Input: part model. Units: mm. Frame: model coordinates. A direction names the side the tool comes from. Round coordinates to 2 decimals unless told otherwise and drop trailing zeros. Order: outer loops, then holes, each group sorted by start corner. A loop starts at its lowest first (then second) coordinate and runs counter-clockwise, first axis right, second up. Notation, with made-up numbers: (68, -32) -> (121, -32) arc R21 cw to (121, -1) -> close; hole circle Ø6 at (66, 63). An arc over 180 degrees is marked (long way). Answer as CSV lines item,"result". Start each with the question number.
1) Access query for faces 4 (the face through (31.056, 27.135, 5.07)), 5 (the face through (-10, -33, 10)), 6 (the face through (5.961, -26.846, 14.058)). Directions: +Z, -Z, +X, -X, +Y, -Y. A direction counts if a zero-diameter tool reaches every point of the face in a straight line with its end or side. Return the directions, or none.
2) Section query D-D, the plane z = 15.5. Output: boundary loops of the cut face in (x, y).
3) First-contact query: P1, Ø12, axis at x = 18, y = -30, coming from the -Z side; P2, Ø5.5, axis at x = 28.28, y = -28.28, coming from the +Z side; P3, Ø7, axis at x = -28.28, y = 28.28, coming from the +Z side; P4, Ø10, axis at y = 4.5, z = 27, coming from the +X side. Flat tips, straight axial feed; report the tip coordinate or a pass-through.
4) Section query A-A, the plane y = 0. State how many separate pieces and enclosed holes the cut face has, and give its area (4 significant figures).
5) Line query: L1, parallel to Z at x = 37.5, y = 18; L2, parallel to X at y = 8, z = 30.5. Output: solid intervals per line, ascending.
6) Mould query, pull axis Y, two halves, no side actions, for faces 1 (the face through (18.28, 28.67, 21.09)), 2 (the face through (0, 43, 5)), 3 (the face through (-1, -29, 0)). Classes: +Y half, -Y half, draft (parallel to the pull), parting line (faces both ways), or undercut.
```python
from build123d import *

# Parameters (mm, degrees)
SKETCH_1_R          = 45
EXTRUDE_1_DEPTH     = 10
SKETCH_2_R          = 34
EXTRUDE_2_DEPTH     = 23
SKETCH_4_R          = 25
CUT_EXTRUDE_1_DEPTH = 70
SKETCH_5_R          = 27.5
CUT_EXTRUDE_2_DEPTH = 28
SKETCH_6_R          = 3
CUT_EXTRUDE_3_DEPTH = 25
CHAMFER_1_SIZE      = 0.5


with BuildPart() as part:
    # 草图1 → 拉伸1 (new body)
    with BuildSketch(Plane.XY):
        Circle(SKETCH_1_R)
    extrude(amount=EXTRUDE_1_DEPTH)

    # 草图2 → 拉伸2 (add)
    with BuildSketch(Plane.XY.offset(10)):
        Circle(SKETCH_2_R)
    extrude(amount=EXTRUDE_2_DEPTH)

    # 草图4 → 切除-拉伸1 (cut)
    with BuildSketch(Plane.XY.offset(33)):
        Circle(SKETCH_4_R)
    extrude(amount=-CUT_EXTRUDE_1_DEPTH, mode=Mode.SUBTRACT)

    # 草图5 → 切除-拉伸2 (cut)
    with BuildSketch(Plane(origin=(0, 0, 0), x_dir=(-1, 0, 0), z_dir=(0, 0, -1))):
        Circle(SKETCH_5_R)
    extrude(amount=-CUT_EXTRUDE_2_DEPTH, mode=Mode.SUBTRACT)

    # 草图6 → 切除-拉伸3 (cut)
    with BuildSketch(Plane.XY.offset(10)):
        with Locations((28.284271247, 28.284271247)):
            Circle(SKETCH_6_R)
        with Locations((40, 0)):
            Circle(SKETCH_6_R)
        with Locations((28.284271247, -28.284271247)):
            Circle(SKETCH_6_R)
        with Locations((0, -40)):
            Circle(SKETCH_6_R)
        with Locations((-28.284271247, -28.284271247)):
            Circle(SKETCH_6_R)
        with Locations((0, 40)):
            Circle(SKETCH_6_R)
        with Locations((-40, 0)):
            Circle(SKETCH_6_R)
        with Locations((-28.284271247, 28.284271247)):
            Circle(SKETCH_6_R)
    extrude(amount=-CUT_EXTRUDE_3_DEPTH, mode=Mode.SUBTRACT)

    # 倒角1
    chamfer_1_edges = [part.edges().sort_by_distance(p)[0] for p in [
        (-25, 0, 33),
        (27.5, 0, 0),
        (-25, 0, 28),
        (-45, 0, 0),
        (-45, 0, 10),
        (-34, 0, 33),
    ]]
    chamfer(chamfer_1_edges, length=CHAMFER_1_SIZE)


solid = part.part
```
Findings:
1,face 4,"+Z, -Z"
1,face 5,"+Z"
1,face 6,"-Z"
2,outline,"circle Ø68 at (0, 0); hole circle Ø55 at (0, 0)"
3,P1,"stops at z = 0"
3,P2,"passes through"
3,P3,"stops at z = 10"
3,P4,"stops at x = 34"
4,separate pieces,"4"
4,enclosed holes,"0"
4,area,"552.5 mm^2"
5,L1,"z = 0 to 10"
5,L2,"x = -33.05 to -23.69, 23.69 to 33.05"
6,face 1,"parting line"
6,face 2,"undercut"
6,face 3,"draft"
